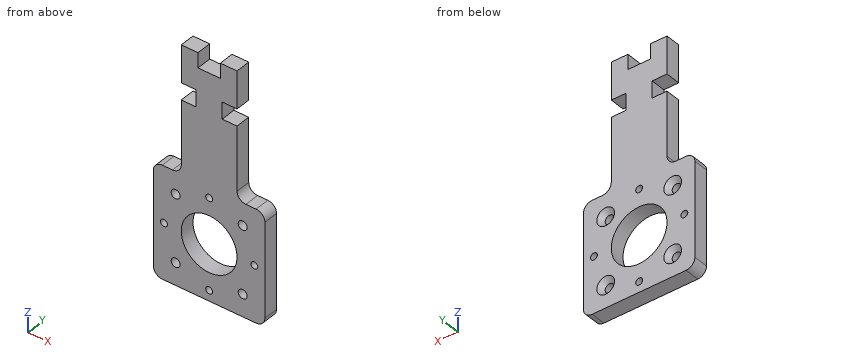
Autodesk Inventor part; units mm, degrees
ref_plane "YZ Plane" through (0, 0, 0) normal (1, 0, 0) x (0, 1, 0)
ref_plane "XZ Plane" through (0, 0, 0) normal (0, 1, 0) x (-1, 0, 0)
ref_plane "XY Plane" through (0, 0, 0) normal (0, 0, 1) x (1, 0, 0)
sketch "Sketch1" plane through (0, 0, 0) normal (0, 1, 0) x (-1, 0, 0)
  line L0 (20, 16.825) -> (20, -16.825)
  line L1 (16.825, -20) -> (-16.825, -20)
  line L2 (-20, -16.825) -> (-20, 16.825)
  line L3 (-16.825, 20) -> (-13.175, 20)
  line L4 (-10, 23.175) -> (-10, 60)
  line L5 (-10, 60) -> (10, 60)
  line L6 (10, 60) -> (10, 23.175)
  line L7 (13.175, 20) -> (16.825, 20)
  arc A0 (10, 23.175) -> (13.175, 20) centre (13.175, 23.175) ccw
  arc A1 (-13.175, 20) -> (-10, 23.175) centre (-13.175, 23.175) ccw
  arc A2 (20, 16.825) -> (16.825, 20) centre (16.825, 16.825) ccw
  arc A3 (16.825, -20) -> (20, -16.825) centre (16.825, -16.825) ccw
  arc A4 (-20, -16.825) -> (-16.825, -20) centre (-16.825, -16.825) ccw
  arc A5 (-16.825, 20) -> (-20, 16.825) centre (-16.825, 16.825) ccw
  point P0 (0, 0)
  point P1 (20, 20)
  point P2 (20, -20)
  point P3 (-20, -20)
  point P4 (-20, 20)
  point P5 (-10, 20)
  point P6 (10, 20)
  point P7 (20, 0)
  point P8 (0, -20)
  point P9 (0, 60)
  dimension "d0" = 40
  dimension "d1" = 40
  dimension "d2" = 20
  dimension "d3" = 60
  dimension "d26" = 3.175
  dimension "d27" = 3.175
extrude "Extrusion1" add sketch "Sketch1" along normal blind 5.334
sketch "Sketch2" plane through (0, 5.334, 0) normal (0, 1, 0) x (1, 0, 0)
  line L0 (-12.0208, -12.0208) -> (0, 0)
  line L1 (0, 0) -> (-20, 0)
  line L2 (-20, 16.825) -> (-20, -16.825)
  point P0 (-17.5, 17.5)
  point P1 (-17.5, -17.5)
  point P2 (12.0208, -12.0208)
  point P3 (12.0208, 12.0208)
  point P4 (-12.0208, 12.0208)
  dimension "d6" = 17
  dimension "d7" = 45
  dimension "d10" = 360
hole "Hole1" at (-12.0208, 5.334, 12.0208) at (12.0208, 5.334, 12.0208) at (12.0208, 5.334, -12.0208) at (-12.0208, 5.334, -12.0208) direction (0, -1, 0) diameter 3.2 end through all countersink diameter 6.35 countersink angle 82
sketch "Sketch3" plane through (0, 5.334, 0) normal (0, 1, 0) x (1, 0, 0)
  point P0 (0, 0)
  point P1 (0, 0)
hole "Hole2" at (0, 5.334, 0) direction (0, -1, 0) diameter 20 end through all
sketch "Sketch4" plane through (0, 5.334, 0) normal (0, 1, 0) x (1, 0, 0)
  point P0 (0, 0)
  point P1 (-16.215, 0)
  point P2 (0, -16.215)
  point P3 (16.215, 0)
  point P4 (0, 16.215)
  dimension "d29" = 16.215
  dimension "d47" = 360
hole "Hole3" at (-16.215, 5.334, 0) at (0, 5.334, 16.215) at (16.215, 5.334, 0) at (0, 5.334, -16.215) direction (0, -1, 0) diameter 2.4638 end through all
sketch "Sketch6" plane through (10, 0, 60) normal (1, 0, 0) x (0, 0, -1)
  line L0 (0, 5.334) -> (36.825, 5.334)
  line L1 (0, 0) -> (36.825, 0)
  line L2 (14, 5.334) -> (8, 5.334)
  line L3 (8, 5.334) -> (8, 0)
  line L4 (8, 0) -> (14, 0)
  line L5 (14, 0) -> (14, 5.334)
  line L6 (0, 0) -> (0, 5.334)
  point P0 (60, 0)
  dimension "d41" = 6
  dimension "d42" = 8
extrude "Extrusion3" cut sketch "Sketch6" against normal blind 5.334 contours L0 L5 L1 L3
sketch "Sketch5" plane through (-10, 0, 60) normal (0, 0, 1) x (1, 0, 0)
  line L0 (26.825, 0) -> (-6.825, 0)
  line L1 (20, 5.334) -> (14, 5.334)
  line L2 (14, 5.334) -> (14, 0)
  line L3 (14, 0) -> (20, 0)
  line L4 (20, 0) -> (20, 5.334)
  line L5 (0, 5.334) -> (20, 5.334)
  line L6 (0, 0) -> (6, 0)
  line L7 (6, 0) -> (6, 5.334)
  line L8 (6, 5.334) -> (0, 5.334)
  line L9 (0, 5.334) -> (0, 0)
  point P0 (10, 0)
  dimension "d37" = 6
  dimension "d38" = 6
extrude "Extrusion2" add sketch "Sketch5" along normal blind 5.334 contours L0 L2 L1 L4 | L0 L9 L5 L7
mirror "Mirror1" about plane through (0, 0, 0) normal (1, 0, 0) of "Extrusion3"
equation "\"d38\" = d37"
properties part number "pitch_mount"
The model under review builds one solid part; all positions refer to its coordinate system, in mm. Give positions to 0.01 mm unless a question says otherwise; leave off trailing zeros. Write each loop counter-clockwise with the first axis right and the second up, starting at its lowest first coordinate (ties: lowest second). Pieces come first, ordered by that corner, then holes.
1. Add section A-A, the plane z = 0. Write out the cut boundary in (x, y).
2. For P1, Ø3, axis at y = 1, z = 46, coming from the -X side; P2, Ø4, axis at x = -12.02, z = 12.02, coming from the +Y side; P3, Ø1.6, axis at y = 2.5, z = 49.5, coming from the +X side, all flat-tipped, find the tip position at first contact; note any pin that passes through.
3. Add section B-B, the plane x = 0. Write out the cut boundary in (y, z).
4. Add section C-C, the plane z = 29. Write out the cut boundary in (x, y).
5. Add section D-D, the plane y = 1.55. Count the separate pieces of the cut face and the enclosed holes in it, plus the area to 3 significant figures.
6. Wall thickness on L1, parallel to Z at x = 0, y = 3.55; L2, parallel to Z at x = 1, y = 4.1; L3, parallel to Z at x = 6, y = 4.7: over which ranges is each line inside the solid? List them lowest first.
Worked answers:
1. outline: (-20, 0) - (-17.45, 0) - (-17.45, 5.33) - (-20, 5.33) - close; (-14.98, 0) - (-10, 0) - (-10, 5.33) - (-14.98, 5.33) - close; (10, 0) - (14.98, 0) - (14.98, 5.33) - (10, 5.33) - close; (17.45, 0) - (20, 0) - (20, 5.33) - (17.45, 5.33) - close
2. P1: stops at x = -10
2. P2: stops at y = 3.98
2. P3: stops at x = 4.67
3. outline: (0, -20) - (5.33, -20) - (5.33, -17.45) - (0, -17.45) - close; (0, -14.98) - (5.33, -14.98) - (5.33, -10) - (0, -10) - close; (0, 10) - (5.33, 10) - (5.33, 14.98) - (0, 14.98) - close; (0, 17.45) - (5.33, 17.45) - (5.33, 60) - (0, 60) - close
4. outline: (-10, 0) - (10, 0) - (10, 5.33) - (-10, 5.33) - close
5. separate pieces: 1
5. enclosed holes: 9
5. area: 2,030 mm2
6. L1: z = -20 to -17.45, -14.98 to -10, 10 to 14.98, 17.45 to 60
6. L2: z = -20 to -16.93, -15.5 to -9.95, 9.95 to 15.5, 16.93 to 60
6. L3: z = -20 to -8, 8 to 46, 52 to 65.33
